Geometry: final body of the model. Coordinates: model frame, mm. Coordinates: 2 decimals unless noted, no trailing zeros. Order: outer loops, then holes, each group sorted by start corner. A loop starts at its lowest first (then second) coordinate and runs counter-clockwise, first axis right, second up. Notation, with made-up numbers: (-17.75, 61.25) -> (-3.75, 61.25) arc R19 ccw to (-3.75, 72.25) -> close; hole circle Ø8 at (42, 17.25). An arc over 180 degrees is marked (long way). Use CSV: the item, a comma, the result in double quotes. Start each with the question number.
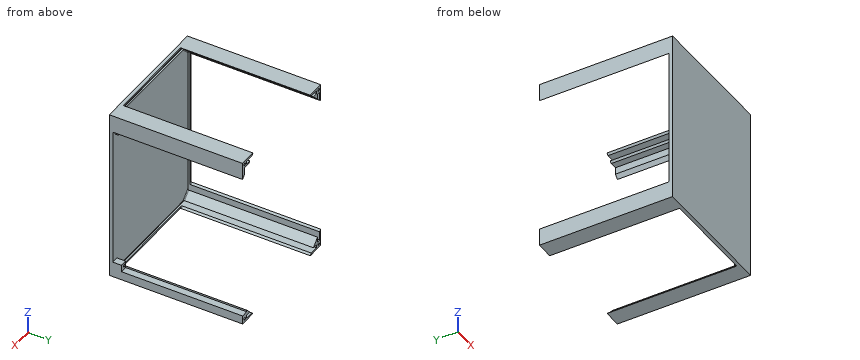
Autodesk Inventor part; units mm, degrees
ref_plane "Pracovní rovina1" through (0, 14, 0) normal (0, 1, 0) x (1, 0, 0)
ref_plane "YZ Plane" through (0, 0, 0) normal (1, 0, 0) x (0, 1, 0)
ref_plane "XZ Plane" through (0, 0, 0) normal (0, 1, 0) x (-1, 0, 0)
sketch "Náčrt1" plane through (0, 0, 0) normal (0, 1, 0) x (-1, 0, 0)
  line L0 (75, 100) -> (-75, 100)
  line L1 (-75, 100) -> (-75, -100)
  line L2 (-75, -100) -> (75, -100)
  line L3 (75, -100) -> (75, 100)
  line L4 (105, 0) -> (-105, 0)
  line L5 (0, -140) -> (0, 140)
  point P0 (0, 0)
  dimension "d0" = 200
  dimension "d1" = 150
extrude "Vysunutí1" add sketch "Náčrt1" along normal blind 4
sketch "Náčrt2" plane through (0, 4, 0) normal (0, 1, 0) x (1, 0, 0)
  line L0 (-75, -100) -> (-75, -80)
  line L1 (-75, -100) -> (-55, -100)
  line L2 (-75, 100) -> (-75, -100)
  line L3 (-75, -100) -> (75, -100)
  line L4 (-69, -86) -> (-69, -92)
  line L5 (-69, -92) -> (-73, -92)
  line L6 (-73, -92) -> (-73, -82)
  line L7 (-73, -82) -> (-75, -80)
  line L8 (-67, -98) -> (-57, -98)
  line L9 (-61, -94) -> (-67, -94)
  line L10 (-67, -94) -> (-67, -98)
  line L11 (-55, -100) -> (-57, -98)
  line L12 (-61, -94) -> (-69, -86)
  point P0 (0, 0)
  dimension "d4" = 20
  dimension "d9" = 2
  dimension "d10" = 4
  dimension "d11" = 10
  dimension "d12" = 6
  dimension "d13" = 8
  dimension "d17" = 4
  dimension "d18" = 2
  dimension "d19" = 8
  dimension "d20" = 10
  dimension "d21" = 6
extrude "Vysunutí2" add sketch "Náčrt2" along normal blind 150
mirror "Zrcadlit1" about plane through (0, 0, 0) normal (0, 0, 1) of "Vysunutí2"
sketch "Náčrt3" plane through (0, 154, 0) normal (0, 1, 0) x (1, 0, 0)
  line L0 (-69, -92) -> (-73, -92)
  line L1 (-67, -98) -> (-67, -94)
  point P0 (0, 0)
  point P1 (-71, -96)
  dimension "d22" = 4
  dimension "d23" = 4
hole "Díra1" at (-71, 154, 96) direction (0, -1, 0) diameter 3 depth 15 tip angle 118
mirror "Zrcadlit2" about plane through (0, 0, 0) normal (0, 0, 1) of "Díra1"
sketch "Náčrt4" plane through (0, 4, 0) normal (0, 1, 0) x (1, 0, 0)
  line L0 (55, -100) -> (75, -100)
  line L1 (75, -100) -> (75, -80)
  line L2 (-55, -100) -> (75, -100)
  line L3 (75, -100) -> (75, 100)
  line L4 (57, -98) -> (67, -98)
  line L5 (67, -98) -> (67, -94)
  line L6 (67, -94) -> (61, -94)
  line L7 (75, -80) -> (61, -94)
  line L8 (57, -98) -> (55, -100)
  point P0 (0, 0)
  dimension "d31" = 20
  dimension "d32" = 20
  dimension "d37" = 10
  dimension "d38" = 6
  dimension "d39" = 8
  dimension "d40" = 2
  dimension "d41" = 45
extrude "Vysunutí3" add sketch "Náčrt4" along normal blind 150
mirror "Zrcadlit3" about plane through (0, 0, 0) normal (0, 0, 1) of "Vysunutí3"
ref_plane "Pracovní rovina1" through (0, 14, 0) normal (0, 1, 0) x (1, 0, 0)
sketch "Náčrt7" plane through (0, 4, 0) normal (0, 1, 0) x (1, 0, 0)
  line L0 (66, -80) -> (71, -80)
  line L1 (71, -80) -> (71, -75)
  line L2 (71, -75) -> (66, -75)
  line L3 (66, -75) -> (66, -80)
  line L4 (75, -80) -> (75, 80)
  line L5 (55, -100) -> (75, -100)
  point P0 (0, 0)
  dimension "d51" = 4
  dimension "d52" = 5
  dimension "d53" = 20
  dimension "d54" = 5
extrude "Vysunutí6" add sketch "Náčrt7" along normal blind 4
mirror "Zrcadlit4" about plane through (0, 0, 0) normal (1, 0, 0) of "Díra1", "Zrcadlit2"
sketch "Náčrt9" plane through (0, 4, 0) normal (0, 1, 0) x (1, 0, 0)
  line L0 (-67, -94) -> (67, -94)
  line L1 (67, -94) -> (67, -98)
  line L2 (67, -98) -> (-67, -98)
  line L3 (-67, -98) -> (-67, -94)
  line L4 (-67, -98) -> (-67, -94)
  line L5 (67, -94) -> (67, -98)
  line L6 (-57, -98) -> (-67, -98)
  line L7 (-67, -94) -> (-61, -94)
  point P0 (0, 0)
extrude "Vysunutí7" cut sketch "Náčrt9" against normal blind 2
mirror "Zrcadlit5" about plane through (0, 0, 0) normal (0, 0, 1) of "Vysunutí7"
sketch "Náčrt10" plane through (0, 4, 0) normal (0, 1, 0) x (1, 0, 0)
  line L0 (-69, -92) -> (-73, -92)
  line L1 (-73, -92) -> (-73, 92)
  line L2 (-73, 92) -> (-69, 92)
  line L3 (-69, 92) -> (-69, -92)
  line L4 (-69, 92) -> (-73, 92)
  line L5 (-69, -92) -> (-73, -92)
  line L6 (-73, -92) -> (-73, -82)
  line L7 (-69, -86) -> (-69, -92)
  point P0 (0, 0)
extrude "Vysunutí8" cut sketch "Náčrt10" against normal blind 2
sketch "Náčrt11" plane through (0, 154, 0) normal (0, 1, 0) x (1, 0, 0)
  line L0 (63, -92) -> (71, -92)
  line L1 (71, -92) -> (71, -84)
  line L2 (71, -84) -> (63, -84)
  line L3 (63, -84) -> (63, -92)
  line L4 (66, -80) -> (71, -80)
  line L5 (75, -80) -> (75, 80)
  line L6 (75, -80) -> (61, -94)
  point P0 (0, 0)
  dimension "d70" = 8
  dimension "d71" = 4
extrude "Vysunutí9" cut sketch "Náčrt11" against normal up to surface (150 mm away)
fillet "Zaoblení1" radius 1 12 edges at (-65, 4, 90) (-56, 4, 99) (-74, 4, 81) (-65, 4, -90) (-74, 4, -81) (-56, 4, -99) (56, 4, -99) (56, 4, 99) (62, 4, 93) (73, 4, 82) (67, 4, 92) (71, 4, 88)
sketch "Náčrt13" plane through (55, 154, -100) normal (0, 1, 0) x (1, 0, 0)
  line L0 (20, -10) -> (12, -10)
  line L1 (12, -10) -> (12, -20)
  line L2 (12, -20) -> (20, -20)
  line L3 (20, -20) -> (20, -10)
  line L4 (20, 0) -> (20, -20)
  point P0 (-55, -100)
  dimension "d78" = 10
  dimension "d79" = 8
extrude "Vysunutí11" cut sketch "Náčrt13" against normal up to surface (150 mm away)
sketch "Náčrt14" plane through (0, 4, 0) normal (0, 1, 0) x (1, 0, 0)
  line L0 (67, 82) -> (75, 82)
  line L1 (75, 82) -> (75, 90)
  line L2 (75, 90) -> (67, 90)
  line L3 (67, 90) -> (67, 82)
  line L4 (67, 88) -> (67, 90)
  line L5 (67, 90) -> (75, 90)
  line L6 (75, -78.5858) -> (75, 90)
  point P0 (0, 0)
  dimension "d82" = 8
extrude "Vysunutí12" add sketch "Náčrt14" along normal blind 10
sketch "Náčrt15" plane through (0, 14, 0) normal (0, 1, 0) x (1, 0, 0)
  line L0 (75, 82) -> (75, 90)
  line L1 (67, 90) -> (75, 90)
  point P0 (0, 0)
  point P1 (69.5, 86)
  dimension "d85" = 5.5
  dimension "d86" = 4
hole "Díra3" at (69.5, 14, -86) direction (0, -1, 0) diameter 3 depth 5
properties part number "Cabinet"
(1) Section C-C (y = 68). State how many separate pieces and enclosed holes the cut face has, then the cut area to 3 significant figures.
(2) Line query: line 1 (X direction, y = 145, z = -96); line 2 (Z direction, x = 69.5, y = 12.5); line 3 (Y direction, x = -14, z = 6). Output: solid intervals per line, ascending. Write a range as from..to.
(3) Section A-A (x = -49.5). Return loops of the section in (y, z).
(4) First-contact query: pin 1 (1.2 mm diameter, centred on x = -70.5, z = 38, fed in from +Y); pin 2 (5.5 mm diameter, centred on x = 67.5, z = 76.5, fed in from +Y); pin 3 (1 mm diameter, centred on x = 20.5, z = -99.5, fed in from +Y). Flat tips, straight axial feed; report the tip coordinate or a pass-through.
(5) Section B-B (z = 57). Return loops of the section in (x, y).
Check sheet entries:
1,separate pieces,"4"
1,enclosed holes,"0"
1,area,"528 mm^2"
2,line 1,"x = -75..-72.5, -69.5..-67, 67..69.5, 72.5..75"
2,line 2,"z = -100..-87.5, -84.5..-82, 92..100"
2,line 3,"y = 0..4"
3,outline,"(0, -100) -> (4, -100) -> (4, -98) -> (2, -98) -> (2, -94) -> (4, -94) -> (4, 94) -> (2, 94) -> (2, 98) -> (4, 98) -> (4, 100) -> (0, 100) -> close"
4,pin 1,"stops at y = 2"
4,pin 2,"stops at y = 8"
4,pin 3,"stops at y = 4"
5,outline,"(-75, 0) -> (75, 0) -> (75, 4) -> (-69, 4) -> (-69, 2) -> (-73, 2) -> (-73, 4) -> (-75, 4) -> close"
